Work out the finished part from the listing and answer in its coordinate system (mm). Face numbers are marked on the shaded views. A direction names the side the tool comes from. Round coordinates to 2 decimals unless told otherwise and drop trailing zeros. Order: outer loops, then holes, each group sorted by start corner. A loop starts at its lowest first (then second) coordinate and runs counter-clockwise, first axis right, second up. Notation, with made-up numbers: (-5, -13.5) - (36, -13.5) arc R10 cw to (36, -0.5) - close; hole circle Ø1 at (29.5, 12.25). An arc over 180 degrees is marked (long way). One line per question, with ' | ' between items. Start each with the question number.
from build123d import *

# Parameters (mm, degrees)
BOSS_EXTRUDE1_DEPTH = 12.7
SKETCH2_W           = 12.7
SKETCH2_H           = 12.7
BOSS_EXTRUDE2_DEPTH = 8.382


with BuildPart() as part:
    # Sketch1 → Boss-Extrude1 (new body)
    with BuildSketch(Plane(origin=(0, 0, 0), x_dir=(1, 0, 0), z_dir=(0, 1, 0))):
        with BuildLine():
            Line((25.4, 0), (88.9, 0))
            ThreePointArc((88.9, 0), (101.6, 12.7), (114.3, 0))
            Line((114.3, 0), (127, 0))
            Line((127, 0), (127, 6.35))
            Line((127, 6.35), (123.597045256, 6.35))
            ThreePointArc((123.597045256, 6.35), (120.422045256, 7.200738686), (118.097783942, 9.525))
            ThreePointArc((118.097783942, 9.525), (101.6, 19.05), (85.102216058, 9.525))
            ThreePointArc((85.102216058, 9.525), (82.777954744, 7.200738686), (79.602954744, 6.35))
            Line((79.602954744, 6.35), (34.697045256, 6.35))
            ThreePointArc((34.697045256, 6.35), (31.522045256, 7.200738686), (29.197783942, 9.525))
            ThreePointArc((29.197783942, 9.525), (12.7, 19.05), (-3.797783942, 9.525))
            ThreePointArc((-3.797783942, 9.525), (-6.122045256, 7.200738686), (-9.297045256, 6.35))
            Line((-9.297045256, 6.35), (-12.7, 6.35))
            Line((-12.7, 6.35), (-12.7, 0))
            Line((-12.7, 0), (0, 0))
            ThreePointArc((0, 0), (12.7, 12.7), (25.4, 0))
        make_face()
    extrude(amount=BOSS_EXTRUDE1_DEPTH)

    # Sketch2 → Boss-Extrude2 (add)
    with BuildSketch(Plane.XY):
        with Locations((-6.35, 6.35)):
            Rectangle(SKETCH2_W, SKETCH2_H)
        with Locations((120.65, 6.35)):
            Rectangle(SKETCH2_W, SKETCH2_H)
    extrude(amount=BOSS_EXTRUDE2_DEPTH)


solid = part.part
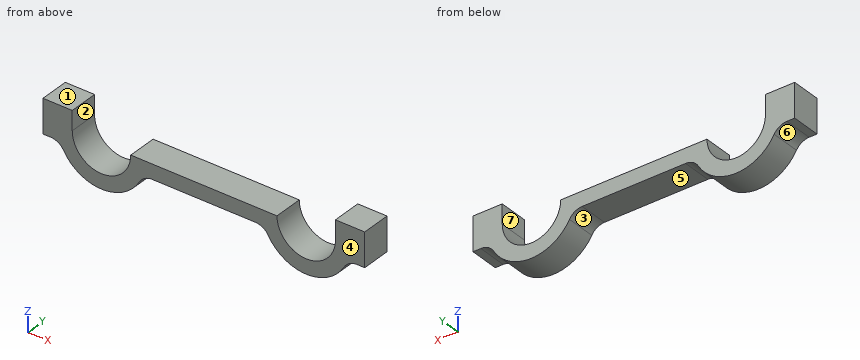
1) Section B-B on y = 11.25 is taken. Give the vertices of the cut face in (x, z) (3 decimals).
2) For the marked faces 1, 2 and 3, determine the directions among +Z, -Z, +X, -X, +Y, -Y from which every point of the face is accessible in a straight line to the end or side of a thin tool.
3) Flat-ended cylindrical pins translate along their axes: pin 1 (6 mm diameter, centred on y = 1.5, z = -7.5, fed in from -X); pin 2 (3 mm diameter, centred on x = 62.5, y = 9, fed in from +Z); pin 3 (6.5 mm diameter, centred on x = 56, y = 9.5, fed in from -Z); pin 4 (1.7 mm diameter, centred on x = 124.5, y = 6.5, fed in from -Z). Find the tip coordinate at first contact, or state that the pin passes through.
4) Section D-D on x = 64 is taken. Give the vertices of the cut face in (y, z), and give its area (3 significant figures).
5) Straight lines are drawn through the part: line 1 (X direction, y = 4.75, z = -0.25); line 2 (X direction, y = 6.25, z = -11.75); line 3 (Z direction, x = 12.5, y = 5). For each, find the intervals that lie inside material, in ascending order.
6) Section A-A on z = 6.25 is taken. Give the vertices of the cut face in (x, y), and give its area (3 significant figures).
7) Determine the mould class of the marked faces 4, 5, 6 and 7 for opening direction X: released by +X, released by -X, zero draft, split by the parting line, or undercut.
8) Section C-C on z = -4 is taken. Give the vertices of the cut face in (x, y).
Recorded:
1) outline: (-12.7, -6.35) - (-9.297, -6.35) arc R6.35 cw to (-3.798, -9.525) arc R19.05 ccw to (29.198, -9.525) arc R6.35 cw to (34.697, -6.35) - (79.603, -6.35) arc R6.35 cw to (85.102, -9.525) arc R19.05 ccw to (118.098, -9.525) arc R6.35 cw to (123.597, -6.35) - (127, -6.35) - (127, 8.382) - (114.3, 8.382) - (114.3, 0) arc R12.7 cw to (88.9, 0) - (25.4, 0) arc R12.7 cw to (0, 0) - (0, 8.382) - (-12.7, 8.382) - close
2) face 1: +Z, +X, -X, +Y, -Y | face 2: +Z, +Y, -Y | face 3: -Z, +Y, -Y
3) pin 1: stops at x = -12.7 | pin 2: stops at z = 0 | pin 3: stops at z = -6.35 | pin 4: stops at z = -6.35
4) outline: (0, -6.35) - (12.7, -6.35) - (12.7, 0) - (0, 0) - close | area: 80.6 mm²
5) line 1: x = -12.7 to 0, 25.4 to 88.9, 114.3 to 127 | line 2: x = -2.29 to 7.88, 17.52 to 27.69, 86.61 to 96.78, 106.42 to 116.59 | line 3: z = -19.05 to -12.7
6) outline: (-12.7, 0) - (0, 0) - (0, 12.7) - (-12.7, 12.7) - close; (114.3, 0) - (127, 0) - (127, 12.7) - (114.3, 12.7) - close | area: 323 mm²
7) face 4: zero draft | face 5: undercut | face 6: released by -X | face 7: undercut
8) outline: (-12.7, 0) - (0.65, 0) - (0.65, 12.7) - (-12.7, 12.7) - close; (24.75, 0) - (89.55, 0) - (89.55, 12.7) - (24.75, 12.7) - close; (113.65, 0) - (127, 0) - (127, 12.7) - (113.65, 12.7) - close
